Could you check a few things on this drawing? It's one solid part, dimensions in mm from its lowest x, y, z. A direction names the side the tool comes from. Give positions to 0.01 mm unless a question says otherwise; leave off trailing zeros. Order: outer loops, then holes, each group sorted by start corner. A loop starts at its lowest first (then second) coordinate and runs counter-clockwise, first axis right, second up.
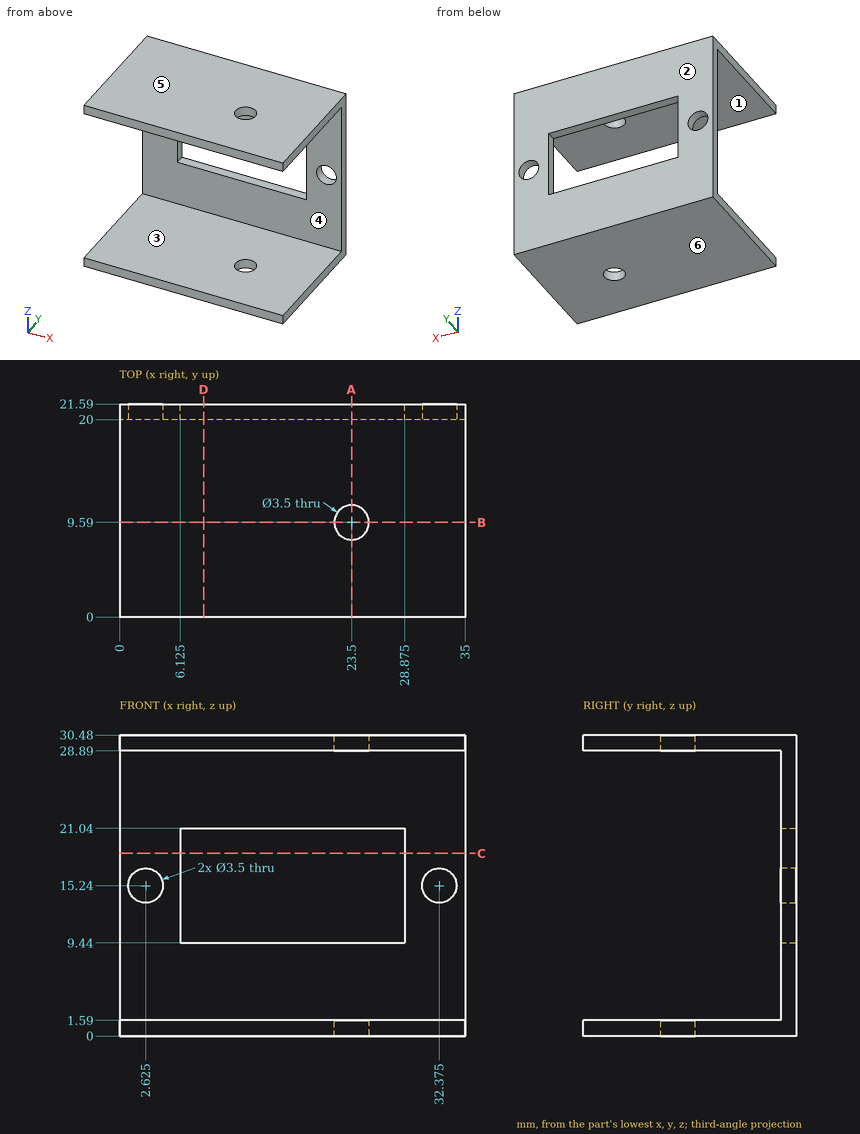
Q1. If we section it at C-C on z = 18.5: List the corners of the cut face in (x, y) for me (3 decimals).
Filled sheet:
outline: (0, 20) - (6.125, 20) - (6.125, 21.59) - (0, 21.59) - close; (28.875, 20) - (35, 20) - (35, 21.59) - (28.875, 21.59) - close
Q2. If we section it at D-D on x = 8.5: List the corners of the cut face in (y, z) for me, plus the area to 3 significant figures.
Filled sheet:
outline: (0, 0) - (21.59, 0) - (21.59, 9.44) - (20, 9.44) - (20, 1.59) - (0, 1.59) - close; (0, 28.89) - (20, 28.89) - (20, 21.04) - (21.59, 21.04) - (21.59, 30.48) - (0, 30.48) - close
area: 93.6 mm2
Q3. Thinking about a two-plate mould opening in Z: for the marked faces 3, 4, 5 and 6, which applies, released by +Z, released by -Z, zero draft, split by the parting line, or undercut?
Filled sheet:
face 3: undercut
face 4: undercut
face 5: released by +Z
face 6: released by -Z
Q4. If we section it at B-B on y = 9.59: List the corners of the cut face in (x, z) for me, plus the area to 3 significant figures.
Filled sheet:
outline: (0, 0) - (21.75, 0) - (21.75, 1.59) - (0, 1.59) - close; (0, 28.89) - (21.75, 28.89) - (21.75, 30.48) - (0, 30.48) - close; (25.25, 0) - (35, 0) - (35, 1.59) - (25.25, 1.59) - close; (25.25, 28.89) - (35, 28.89) - (35, 30.48) - (25.25, 30.48) - close
area: 100 mm2
Q5. If we section it at A-A on x = 23.5: List the corners of the cut face in (y, z) for me, plus the area to 3 significant figures.
Filled sheet:
outline: (0, 0) - (7.84, 0) - (7.84, 1.59) - (0, 1.59) - close; (0, 28.89) - (7.84, 28.89) - (7.84, 30.48) - (0, 30.48) - close; (11.34, 0) - (21.59, 0) - (21.59, 9.44) - (20, 9.44) - (20, 1.59) - (11.34, 1.59) - close; (11.34, 28.89) - (20, 28.89) - (20, 21.04) - (21.59, 21.04) - (21.59, 30.48) - (11.34, 30.48) - close
area: 82.5 mm2
Q6. I'm going to push a flat-ended pin straight in: P1, Ø1, axis at x = 28.5, z = 8, coming from the -Y side. Where does the tip first touch, or does it pass through?
Filled sheet:
P1: stops at y = 20
Q7. I need wall thicknesses on L1, parallel to X at y = 21.15, z = 15.24 (3 decimals); L2, parallel to Y at x = 23.5, z = 1; L3, parallel to Z at x = 32.5, y = 12.5. Which ranges of each line are inside material? Lowest first, please.
Filled sheet:
L1: x = 0 to 0.875, 4.375 to 6.125, 28.875 to 30.625, 34.125 to 35
L2: y = 0 to 7.84, 11.34 to 21.59
L3: z = 0 to 1.59, 28.89 to 30.48
Q8. For the marked faces 1 and 2, which set-ups out of +Z, -Z, +X, -X, +Y, -Y let a thin tool reach every point of the face, with its end or its side?
Filled sheet:
face 1: +X, -X, -Y
face 2: +Z, -Z, +X, -X, +Y
